The listing builds one solid part. Answer for the finished solid, in the listing's coordinates (mm). A direction names the side the tool comes from. Round coordinates to 2 decimals unless told otherwise and drop trailing zeros. Loops run counter-clockwise (first coordinate to the right, second up) from the corner with the lowest first, then second, coordinate; pieces in that order, holes last. Notation, with made-up numbers: (-15.75, -2.75) -> (-4.75, -2.75) arc R17 ccw to (-4.75, 12.25) -> close; hole circle Ø8 at (77, -18). An arc over 180 degrees is marked (long way). Write each question's results on one line, items separated by ' | '. Start each with the question number.
from build123d import *

# Parameters (mm, degrees)
SKETCH1_R           = 44.5
BOSS_EXTRUDE1_DEPTH = 12
SKETCH3_R           = 44.5
SKETCH3_R_2         = 42
CUT_EXTRUDE1_DEPTH  = 6
SKETCH4_R           = 17.5
CUT_EXTRUDE2_DEPTH  = 3


with BuildPart() as part:
    # Sketch1 → Boss-Extrude1 (new body)
    with BuildSketch(Plane(origin=(0, 0, 0), x_dir=(0, 0, -1), z_dir=(1, 0, 0))):
        Circle(SKETCH1_R)
    extrude(amount=BOSS_EXTRUDE1_DEPTH)

    # Sketch3 → Cut-Extrude1 (cut)
    with BuildSketch(Plane(origin=(3, 0, 0), x_dir=(0, 0, -1), z_dir=(1, 0, 0))):
        Circle(SKETCH3_R)
        Circle(SKETCH3_R_2, mode=Mode.SUBTRACT)
    extrude(amount=CUT_EXTRUDE1_DEPTH, mode=Mode.SUBTRACT)

    # Sketch4 → Cut-Extrude2 (cut)
    with BuildSketch(Plane.ZY):
        Circle(SKETCH4_R)
    extrude(amount=-CUT_EXTRUDE2_DEPTH, mode=Mode.SUBTRACT)


solid = part.part
Item 1: Straight lines are drawn through the part: L1, parallel to Y at x = 2.35, z = 0; L2, parallel to Y at x = 4, z = -1; L3, parallel to Z at x = 10, y = 8 (3 decimals). For each, find the intervals that lie inside material, in ascending order. Write a range as [from, to].
Item 2: The part is cut by section C-C, the plane x = 7.25. Give the vertices of the cut face in (y, z), plus the area to 3 significant figures.
Item 3: For faces 1 (the flat face through (3, -33, 27)), 2 (the flat face through (3, 0, 0)), 3 (the cylindrical face through (10.479, 30.075, 32.798)), determine the directions among +Z, -Z, +X, -X, +Y, -Y from which every point of the face is accessible in a straight line to the end or side of a thin tool.
Item 4: Determine the mould class of faces 4 (the cylindrical face through (1.479, 30.075, 32.798)), 5 (the cylindrical face through (1.479, -10.648, -13.887)), 6 (the flat face through (9, -33, 27)) for opening direction Z: +Z half, -Z half, draft (parallel to the pull), parting line (faces both ways), or undercut.
Item 5: The part is cut by section A-A, the plane y = 0. Give the vertices of the cut face in (x, z), plus the area to 3 significant figures.
Item 6: The part is cut by section D-D, the plane x = 1.25. Give the vertices of the cut face in (y, z).
Item 7: Each of these flat-tipped pins is pushed along its axis until it touches: pin 1 Ø6 at (x, z) = (3, -13.5) entering from +Y; pin 2 Ø12 at (y, z) = (14, 32.5) entering from -X; pin 3 Ø1 at (x, z) = (2, -13) entering from +Y; pin 4 Ø2 at (x, z) = (8.5, 8.5) entering from +Y. Where does it stop, or does it pass through?
Report:
1) L1: y = [-44.5, -17.5], [17.5, 44.5] | L2: y = [-41.99, 41.99] | L3: z = [-43.775, 43.775]
2) outline: circle Ø84 at (0, 0) | area: 5,540 mm2
3) face 1: none | face 2: -X | face 3: +X, -X
4) face 4: parting line | face 5: undercut | face 6: draft
5) outline: (0, -44.5) -> (3, -44.5) -> (3, -42) -> (9, -42) -> (9, -44.5) -> (12, -44.5) -> (12, 44.5) -> (9, 44.5) -> (9, 42) -> (3, 42) -> (3, 44.5) -> (0, 44.5) -> (0, 17.5) -> (3, 17.5) -> (3, -17.5) -> (0, -17.5) -> close | area: 933 mm2
6) outline: circle Ø89 at (0, 0); hole circle Ø35 at (0, 0)
7) pin 1: stops at y = 43.24 | pin 2: stops at x = 0 | pin 3: stops at y = 42.71 | pin 4: stops at y = 43.84
